For this review, take the finished solid that the model builds, in its own axes (mm). A direction names the side the tool comes from. Round coordinates to 2 decimals unless told otherwise and drop trailing zeros. Loops run counter-clockwise (first coordinate to the right, second up) from the corner with the lowest first, then second, coordinate; pieces in that order, holes last. Notation, with made-up numbers: (49.5, -10.5) -> (107.5, -10.5) arc R35 cw to (107.5, 25.5) -> close; hole circle Ø1 at (49.5, -30.5). An arc over 180 degrees is marked (long way). Write each question's results on one line, items separated by ' | '.
```python
from build123d import *

# Parameters (mm, degrees)
MAIN_EXTRUDE_DEPTH = 40
CUT_EXTRUDE1_START = -4
SKETCH4_W          = 47.4
SKETCH4_H          = 20
CUT_EXTRUDE1_DEPTH = 4
FILLET1_R          = 1
FILLET2_R          = 1
FILLET3_R          = 1


with BuildPart() as part:
    # Sketch1 → Main-Extrude (new body)
    with BuildSketch(Plane(origin=(0, 0, 0), x_dir=(1, 0, 0), z_dir=(0, 1, 0))):
        with BuildLine():
            Line((6.5, 10.159541063), (6.5, 7.17778828))
            ThreePointArc((6.5, 7.17778828), (6.779616102, 6.728977699), (7.305723751, 6.782145779))
            Line((7.305723751, 6.782145779), (11.611447501, 10.10929595))
            ThreePointArc((11.611447501, 10.10929595), (11.897621162, 10.459813156), (12, 10.900580951))
            Line((12, 10.900580951), (12, 15.918501174))
            ThreePointArc((12, 15.918501174), (11.897621162, 16.35926897), (11.611447501, 16.709786176))
            Line((11.611447501, 16.709786176), (7.305723751, 20.036936346))
            ThreePointArc((7.305723751, 20.036936346), (6.779616102, 20.090104427), (6.5, 19.641293846))
            Line((6.5, 19.641293846), (6.5, 16.609541063))
            Line((6.5, 16.609541063), (3, 16.609541063))
            Line((3, 16.609541063), (3, 26.109541063))
            Line((3, 26.109541063), (-1, 26.109541063))
            Line((-1, 26.109541063), (-1, 0.659541063))
            Line((-1, 0.659541063), (-19, 0.659541063))
            Line((-19, 0.659541063), (-19, -3.340458937))
            Line((-19, -3.340458937), (-4.999912017, -3.340458937))
            Line((-4.999912017, -3.340458937), (28.4, -3.340458937))
            Line((28.4, -3.340458937), (28.4, 0.659541063))
            Line((28.4, 0.659541063), (3, 0.659541063))
            Line((3, 0.659541063), (3, 10.159541063))
            Line((3, 10.159541063), (6.5, 10.159541063))
        make_face()
    extrude(amount=MAIN_EXTRUDE_DEPTH)

    # Sketch4 → Cut-Extrude1 (cut)
    with BuildSketch(Plane.XY.offset(3.340458937).offset(CUT_EXTRUDE1_START)):
        with Locations((4.7, 30)):
            Rectangle(SKETCH4_W, SKETCH4_H)
    extrude(amount=CUT_EXTRUDE1_DEPTH, mode=Mode.SUBTRACT)

    # Fillet1
    fillet1_edges = [part.edges().sort_by_distance(p)[0] for p in [
        (28.4, 10, 3.340458937),
        (-19, 10, 3.340458937),
        (28.4, 10, -0.659541063),
    ]]
    fillet(fillet1_edges, radius=FILLET1_R)

    # Fillet2
    fillet2_edges = [part.edges().sort_by_distance(p)[0] for p in [
        (-19, 10, -0.659541063),
    ]]
    fillet(fillet2_edges, radius=FILLET2_R)

    # Fillet3
    fillet3_edges = [part.edges().sort_by_distance(p)[0] for p in [
        (-1, 10, -0.659541063),
    ]]
    fillet(fillet3_edges, radius=FILLET3_R)


solid = part.part
```
1. For pin 1 (5 mm diameter, centred on y = 23.5, z = -22, fed in from +X); pin 2 (1.5 mm diameter, centred on y = 26.5, z = -13, fed in from +X); pin 3 (1 mm diameter, centred on x = 4.5, y = 21, fed in from -Z), all flat-tipped, find the tip position at first contact; note any pin that passes through.
Values found:
pin 1: stops at x = 8 | pin 2: stops at x = 12 | pin 3: stops at z = -16.61
2. Consider section A-A (y = 6.5). State the section outline as (x, z) points, plus the area to 3 significant figures.
Values found:
outline: (-19, 0.34) arc R1 ccw to (-18, -0.66) -> (-2, -0.66) arc R1 cw to (-1, -1.66) -> (-1, -26.11) -> (3, -26.11) -> (3, -16.61) -> (6.5, -16.61) -> (6.5, -19.64) arc R0.5 ccw to (7.31, -20.04) -> (11.61, -16.71) arc R1 ccw to (12, -15.92) -> (12, -10.9) arc R1 ccw to (11.61, -10.11) -> (7.31, -6.78) arc R0.5 ccw to (6.5, -7.18) -> (6.5, -10.16) -> (3, -10.16) -> (3, -0.66) -> (27.4, -0.66) arc R1 ccw to (28.4, 0.34) -> (28.4, 2.34) arc R1 ccw to (27.4, 3.34) -> (-18, 3.34) arc R1 ccw to (-19, 2.34) -> close | area: 369 mm2
3. Consider section C-C (x = 8). State the section outline as (y, z) points.
Values found:
outline: (0, -19.5) -> (40, -19.5) -> (40, -7.32) -> (0, -7.32) -> close; (0, -0.66) -> (20, -0.66) -> (20, 3.34) -> (0, 3.34) -> close
4. Tool access review of faces 5 (the face through (3, 20, -21)), 6 (the face through (3, 20, -5)), 7 (the face through (9.4, 19.7, -8.4)): name each direction out of +Z, -Z, +X, -X, +Y, -Y from which nothing blocks a thin tool from reaching the whole face with its end or side.
Values found:
face 5: -Z, +Y, -Y | face 6: +Y, -Y | face 7: +X, +Y, -Y
5. Consider section B-B (z = -18.75). State the section outline as (x, y) points.
Values found:
outline: (-1, 0) -> (3, 0) -> (3, 40) -> (-1, 40) -> close; (6.5, 0) -> (8.97, 0) -> (8.97, 40) -> (6.5, 40) -> close
6. To check wall thickness, follow probe 1 along Z at (x, y) = (3.5, 8.5); probe 2 along X at (y, z) = (37.5, -14.5); probe 3 along X at (y, z) = (20.5, -9.75). State the ranges of each line that lie inside material, in increasing order.
Values found:
probe 1: z = -16.61 to -10.16, -0.66 to 3.34 | probe 2: x = -1 to 12 | probe 3: x = -1 to 3, 6.5 to 11.15
7. Draft analysis for pull direction X (two halves, no side actions). For faces 1 (the face through (28.4, 10, 1)), 2 (the face through (5, 20, -16.61)), 3 (the face through (6.5, 20, -18)), 4 (the face through (2.8, 0, -7.1)), state which applies: released by +X, released by -X, zero draft, split by the parting line, or undercut.
Values found:
face 1: released by +X | face 2: undercut | face 3: undercut | face 4: zero draft
8. Consider section D-D (x = 21). State the section outline as (y, z) points.
Values found:
outline: (0, -0.66) -> (20, -0.66) -> (20, 3.34) -> (0, 3.34) -> close
